```python
from build123d import *
from build123d.topology import SkipClean

# Parameters (mm, degrees)
CUT_EXTRUDE1_REACH               = 90.75
SKETCH2_R                        = 2
SKETCH2_R_2                      = 1
CUT_EXTRUDE2_REACH               = 90.75
F_18_0_1695_DIAMETER_HOLE1_D     = 4.3053
F_18_0_1695_DIAMETER_HOLE1_DEPTH = 12
CUT_EXTRUDE3_DEPTH               = 28


with BuildPart() as part:
    # Sketch1 → Revolve1 (revolve)
    with BuildSketch(Plane.XY, mode=Mode.PRIVATE) as revolve1_sk:
        Polygon((0, 0), (62.5, 0), (62.5, 12), (50, 12), (50, 4), (0, 4), align=None)
    revolve(revolve1_sk.sketch.rotate(Axis((0, 0, 0), (0, 1, 0)), 90), axis=Axis((0, 0, 0), (0, 1, 0)))

    # Sketch2 → Cut-Extrude1 (cut, up to next)
    with BuildSketch(Plane(origin=(0, 4, 0), x_dir=(1, 0, 0), z_dir=(0, 1, 0)), mode=Mode.PRIVATE) as cut_extrude1_sk1:
        with Locations(Location((0, 0, 0), (0, 0, 270))):
            Circle(SKETCH2_R)
    cut_extrude1_tool1 = extrude(cut_extrude1_sk1.sketch, amount=-CUT_EXTRUDE1_REACH, mode=Mode.PRIVATE) & part.part
    # Sketch2 → Cut-Extrude1 (cut, up to next)
    with BuildSketch(Plane(origin=(0, 4, 0), x_dir=(1, 0, 0), z_dir=(0, 1, 0)), mode=Mode.PRIVATE) as cut_extrude1_sk2:
        with Locations(Location((6.540737726, -6.540737726, 0), (0, 0, 270))):
            Circle(SKETCH2_R_2)
    cut_extrude1_tool2 = extrude(cut_extrude1_sk2.sketch, amount=-CUT_EXTRUDE1_REACH, mode=Mode.PRIVATE) & part.part
    # Sketch2 → Cut-Extrude1 (cut, up to next)
    with BuildSketch(Plane(origin=(0, 4, 0), x_dir=(1, 0, 0), z_dir=(0, 1, 0)), mode=Mode.PRIVATE) as cut_extrude1_sk3:
        with Locations(Location((-6.540737726, 6.540737726, 0), (0, 0, 270))):
            Circle(SKETCH2_R_2)
    cut_extrude1_tool3 = extrude(cut_extrude1_sk3.sketch, amount=-CUT_EXTRUDE1_REACH, mode=Mode.PRIVATE) & part.part
    add(cut_extrude1_tool1.solids().sort_by_distance((0, 4, 0))[0], mode=Mode.SUBTRACT)
    add(cut_extrude1_tool2.solids().sort_by_distance((6.540738, 4, 6.540738))[0], mode=Mode.SUBTRACT)
    add(cut_extrude1_tool3.solids().sort_by_distance((-6.540738, 4, -6.540738))[0], mode=Mode.SUBTRACT)

    # Sketch3 → Cut-Extrude2 (cut, up to next)
    with BuildSketch(Plane(origin=(0, 4, 0), x_dir=(1, 0, 0), z_dir=(0, 1, 0)), mode=Mode.PRIVATE) as cut_extrude2_sk1:
        with BuildLine():
            ThreePointArc((48.869672579, 10.571428571), (35.355339059, 35.355339059), (10.571428571, 48.869672579))
            ThreePointArc((10.571428571, 48.869672579), (3.141290928, 44.082392078), (7.928571429, 36.652254434))
            ThreePointArc((7.928571429, 36.652254434), (26.516504294, 26.516504294), (36.652254434, 7.928571429))
            ThreePointArc((36.652254434, 7.928571429), (44.082392078, 3.141290928), (48.869672579, 10.571428571))
        make_face()
    cut_extrude2_tool1 = extrude(cut_extrude2_sk1.sketch, amount=-CUT_EXTRUDE2_REACH, mode=Mode.PRIVATE) & part.part
    # Sketch3 → Cut-Extrude2 (cut, up to next)
    with BuildSketch(Plane(origin=(0, 4, 0), x_dir=(1, 0, 0), z_dir=(0, 1, 0)), mode=Mode.PRIVATE) as cut_extrude2_sk2:
        with BuildLine():
            ThreePointArc((-48.869672579, 10.571428571), (-35.355339059, 35.355339059), (-10.571428571, 48.869672579))
            ThreePointArc((-10.571428571, 48.869672579), (-3.141290928, 44.082392078), (-7.928571429, 36.652254434))
            ThreePointArc((-7.928571429, 36.652254434), (-26.516504294, 26.516504294), (-36.652254434, 7.928571429))
            ThreePointArc((-36.652254434, 7.928571429), (-44.082392078, 3.141290928), (-48.869672579, 10.571428571))
        make_face()
    cut_extrude2_tool2 = extrude(cut_extrude2_sk2.sketch, amount=-CUT_EXTRUDE2_REACH, mode=Mode.PRIVATE) & part.part
    # Sketch3 → Cut-Extrude2 (cut, up to next)
    with BuildSketch(Plane(origin=(0, 4, 0), x_dir=(1, 0, 0), z_dir=(0, 1, 0)), mode=Mode.PRIVATE) as cut_extrude2_sk3:
        with BuildLine():
            ThreePointArc((48.869672579, -10.571428571), (35.355339059, -35.355339059), (10.571428571, -48.869672579))
            ThreePointArc((10.571428571, -48.869672579), (3.141290928, -44.082392078), (7.928571429, -36.652254434))
            ThreePointArc((7.928571429, -36.652254434), (26.516504294, -26.516504294), (36.652254434, -7.928571429))
            ThreePointArc((36.652254434, -7.928571429), (44.082392078, -3.141290928), (48.869672579, -10.571428571))
        make_face()
    cut_extrude2_tool3 = extrude(cut_extrude2_sk3.sketch, amount=-CUT_EXTRUDE2_REACH, mode=Mode.PRIVATE) & part.part
    # Sketch3 → Cut-Extrude2 (cut, up to next)
    with BuildSketch(Plane(origin=(0, 4, 0), x_dir=(1, 0, 0), z_dir=(0, 1, 0)), mode=Mode.PRIVATE) as cut_extrude2_sk4:
        with BuildLine():
            ThreePointArc((-48.869672579, -10.571428571), (-35.355339059, -35.355339059), (-10.571428571, -48.869672579))
            ThreePointArc((-10.571428571, -48.869672579), (-3.141290928, -44.082392078), (-7.928571429, -36.652254434))
            ThreePointArc((-7.928571429, -36.652254434), (-26.516504294, -26.516504294), (-36.652254434, -7.928571429))
            ThreePointArc((-36.652254434, -7.928571429), (-44.082392078, -3.141290928), (-48.869672579, -10.571428571))
        make_face()
    cut_extrude2_tool4 = extrude(cut_extrude2_sk4.sketch, amount=-CUT_EXTRUDE2_REACH, mode=Mode.PRIVATE) & part.part
    add(cut_extrude2_tool1.solids().sort_by_distance((28.738526, 4, -28.738526))[0], mode=Mode.SUBTRACT)
    add(cut_extrude2_tool2.solids().sort_by_distance((-28.738526, 4, -28.738526))[0], mode=Mode.SUBTRACT)
    add(cut_extrude2_tool3.solids().sort_by_distance((28.738526, 4, 28.738526))[0], mode=Mode.SUBTRACT)
    add(cut_extrude2_tool4.solids().sort_by_distance((-28.738526, 4, 28.738526))[0], mode=Mode.SUBTRACT)

    # #18 (0.1695) Diameter Hole1
    with Locations(Plane(origin=(0, 12, 0), x_dir=(1, 0, 0), z_dir=(0, 1, 0))):
        with Locations((0, 56.25), (56.25, 0), (0, -56.25), (-56.25, 0), (0, 0)):
            Hole(F_18_0_1695_DIAMETER_HOLE1_D / 2, depth=F_18_0_1695_DIAMETER_HOLE1_DEPTH)

    # Sketch6 → Cut-Extrude3 (cut)
    with SkipClean():  # the faces are left unmerged after this step: merging them gives an invalid solid
        with BuildSketch(Plane(origin=(0, 19.982495649, 0), x_dir=(1, 0, 0), z_dir=(0, 1, 0))):
            with BuildLine():
                Line((-56.597564395, 7.921), (-59.13485528, 7.921))
                ThreePointArc((-59.13485528, 7.921), (-61.28824505, 7.07913898), (-62.299678972, 5))
                ThreePointArc((-62.299678972, 5), (-44.194173824, 44.194173824), (-5, 62.299678972))
                ThreePointArc((-5, 62.299678972), (-7.07913898, 61.28824505), (-7.921, 59.13485528))
                Line((-7.921, 59.13485528), (-7.921, 56.597564395))
                ThreePointArc((-7.921, 56.597564395), (-8.64446813, 54.579988512), (-10.485166883, 53.48187801))
                ThreePointArc((-10.485166883, 53.48187801), (-38.537319575, 38.537319575), (-53.48187801, 10.485166883))
                ThreePointArc((-53.48187801, 10.485166883), (-54.579988512, 8.64446813), (-56.597564395, 7.921))
            make_face()
            with BuildLine():
                Line((7.921, 56.597564395), (7.921, 59.13485528))
                ThreePointArc((7.921, 59.13485528), (7.07913898, 61.28824505), (5, 62.299678972))
                ThreePointArc((5, 62.299678972), (44.194173824, 44.194173824), (62.299678972, 5))
                ThreePointArc((62.299678972, 5), (61.28824505, 7.07913898), (59.13485528, 7.921))
                Line((59.13485528, 7.921), (56.597564395, 7.921))
                ThreePointArc((56.597564395, 7.921), (54.579988512, 8.64446813), (53.48187801, 10.485166883))
                ThreePointArc((53.48187801, 10.485166883), (38.537319575, 38.537319575), (10.485166883, 53.48187801))
                ThreePointArc((10.485166883, 53.48187801), (8.64446813, 54.579988512), (7.921, 56.597564395))
            make_face()
            with BuildLine():
                Line((56.597564395, -7.921), (59.13485528, -7.921))
                ThreePointArc((59.13485528, -7.921), (61.28824505, -7.07913898), (62.299678972, -5))
                ThreePointArc((62.299678972, -5), (44.194173824, -44.194173824), (5, -62.299678972))
                ThreePointArc((5, -62.299678972), (7.07913898, -61.28824505), (7.921, -59.13485528))
                Line((7.921, -59.13485528), (7.921, -56.597564395))
                ThreePointArc((7.921, -56.597564395), (8.64446813, -54.579988512), (10.485166883, -53.48187801))
                ThreePointArc((10.485166883, -53.48187801), (38.537319575, -38.537319575), (53.48187801, -10.485166883))
                ThreePointArc((53.48187801, -10.485166883), (54.579988512, -8.64446813), (56.597564395, -7.921))
            make_face()
            with BuildLine():
                Line((-7.921, -56.597564395), (-7.921, -59.13485528))
                ThreePointArc((-7.921, -59.13485528), (-7.07913898, -61.28824505), (-5, -62.299678972))
                ThreePointArc((-5, -62.299678972), (-44.194173824, -44.194173824), (-62.299678972, -5))
                ThreePointArc((-62.299678972, -5), (-61.28824505, -7.07913898), (-59.13485528, -7.921))
                Line((-59.13485528, -7.921), (-56.597564395, -7.921))
                ThreePointArc((-56.597564395, -7.921), (-54.579988512, -8.64446813), (-53.48187801, -10.485166883))
                ThreePointArc((-53.48187801, -10.485166883), (-38.537319575, -38.537319575), (-10.485166883, -53.48187801))
                ThreePointArc((-10.485166883, -53.48187801), (-8.64446813, -54.579988512), (-7.921, -56.597564395))
            make_face()
        extrude(amount=-CUT_EXTRUDE3_DEPTH, mode=Mode.SUBTRACT)


solid = part.part
```
The listing builds one solid part. Answer for the finished solid, in the listing's coordinates (mm). A direction names the side the tool comes from. Coordinates: 2 decimals unless noted, no trailing zeros. Write each loop counter-clockwise with the first axis right and the second up, starting at its lowest first coordinate (ties: lowest second). Pieces come first, ordered by that corner, then holes. Notation, with made-up numbers: (27.25, 65.25) - (85.25, 65.25) arc R19 cw to (85.25, 88.25) - close; hole circle Ø7 at (25.25, 51.25). An arc over 180 degrees is marked (long way). Return JSON: item names as keys, results as strings. Group by question number.
Q1. Which of the six approach directions +Z, -Z, +X, -X, +Y, -Y give full straight-line access (tool end or side, diameter ignored) to faces 5 (the cylindrical face through (0.1, 6.1, -62.5)), 6 (the cylindrical face through (43.948, 2.028, 3.114))?
Q2. The part is cut by section A-A on z = 0. Write down the section's boundary in (x, y), and give its area (3 significant figures).
Q3. Flat-ended cylindrical pins translate along their axes: pin 1 Ø6 at (x, y) = (16.5, 10.5) entering from -Z; pin 2 Ø2.5 at (x, z) = (6.54, 6.54) entering from +Y; pin 3 Ø1.3 at (x, y) = (-57.5, 7.5) entering from +Z. Find the tip coordinate at first contact, or state that the pin passes through.
Q4. For a pull along X with two mould halves and no side action, classify faces 1 (the cylindrical face through (0.47, 5.92, 58.35)), 2 (the cylindrical face through (54.6, 6.08, -8.63)), 3 (the cylindrical face through (-0.1, 6.1, 62.5)), 4 (the cylindrical face through (-8.63, 6.08, -54.6)) as +X half, -X half, draft (parallel to the pull), parting line (faces both ways), or undercut.
Q5. The part is cut by section C-C on z = 25. Write down the section's boundary in (x, y).
Q6. The part is cut by section B-B on x = 40.5. Write down the section's boundary in (y, z).
Q7. Find the intervals of material crossed by line 1 along X through (y, z) = (2.5, 27); line 2 along X through (y, z) = (3.25, 41.5); line 3 along Z through (x, y) = (-13.5, 2), in increasing order. Write a range as [from, to].
Q8. The part is cut by section D-D on y = 10. State how many separate pieces and enclosed holes the cut face has, and give its area (3 significant figures).
Evaluation:
{
 "1": {"face 5": "-Z, +Y, -Y", "face 6": "+Y, -Y"},
 "2": {"outline": "(-62.5, 0) - (-58.4, 0) - (-58.4, 12) - (-62.5, 12) - close; (-54.1, 0) - (-2.15, 0) - (-2.15, 4) - (-50, 4) - (-50, 12) - (-54.1, 12) - close; (2.15, 0) - (54.1, 0) - (54.1, 12) - (50, 12) - (50, 4) - (2.15, 4) - close; (58.4, 0) - (62.5, 0) - (62.5, 12) - (58.4, 12) - close", "area": "579 mm2"},
 "3": {"pin 1": "stops at z = -52.8", "pin 2": "stops at y = 4", "pin 3": "stops at z = 7.92"},
 "4": {"face 1": "undercut", "face 2": "+X half", "face 3": "parting line", "face 4": "-X half"},
 "5": {"outline": "(-48.43, 0) - (-43.3, 0) - (-43.3, 12) - (-48.43, 12) - close; (-27.95, 0) - (27.95, 0) - (27.95, 4) - (-27.95, 4) - close; (43.3, 0) - (48.43, 0) - (48.43, 12) - (43.3, 12) - close"},
 "6": {"outline": "(0, -36.47) - (12, -36.47) - (12, -29.32) - (0, -29.32) - close; (0, -3.42) - (4, -3.42) - (4, 3.42) - (0, 3.42) - close; (0, 29.32) - (12, 29.32) - (12, 36.47) - (0, 36.47) - close"},
 "7": {"line 1": "x = [-47.34, -42.08], [-26.02, 26.02], [42.08, 47.34]", "line 2": "x = [-35.33, -27.89], [-3.13, 3.13], [27.89, 35.33]", "line 3": "z = [-52.8, -48.14], [-34.99, 34.99], [48.14, 52.8]"},
 "8": {"separate pieces": "1", "enclosed holes": "5", "area": "1,930 mm2"}
}
